Here's how the part is built. I have some questions about the finished solid (model axes, mm). Give positions to 0.01 mm unless a question says otherwise; leave off trailing zeros. Use one line per item in the form item = value.
from build123d import *

# Parameters (mm, degrees)
BOSS_EXTRUDE1_DEPTH  = 3.000000026
SKETCH2_R            = 2.767129072
SKETCH2_R_2          = 3.006829377
BOSS_EXTRUDE2_DEPTH  = 3
M3_CLEARANCE_HOLE1_D = 3.2


with BuildPart() as part:
    # Sketch1 → Boss-Extrude1 (new body)
    with BuildSketch(Plane.XZ):
        Polygon((3.305407241, 0.060769264), (3.999999724, 0), (34.000001848, 0), (34.694589674, 0.060769264), (35.368077457, 0.241229776), (35.99999845, 0.535898609), (36.571152508, 0.935822492), (37.064179778, 1.428849762), (37.464100868, 2.000000095), (37.758767605, 2.631919459), (37.939228117, 3.305407474), (37.999998778, 4.00000019), (37.939228117, 4.694593139), (37.758767605, 5.368080921), (37.464100868, 6.000000052), (37.064179778, 6.571150385), (36.571152508, 7.064177655), (35.99999845, 7.464101538), (35.368077457, 7.758770604), (34.694589674, 7.939230651), (34.000001848, 8.00000038), (3.999999724, 8.00000038), (3.305407241, 7.939230651), (2.631919459, 7.758770604), (1.999998465, 7.464101538), (1.428848132, 7.064177655), (0.935820863, 6.571150385), (0.535897911, 6.000000052), (0.241229311, 5.368080921), (0.060768798, 4.694593139), (0, 4.00000019), (0.060768798, 3.305407474), (0.241229311, 2.631919459), (0.535897911, 2.000000095), (0.935820863, 1.428849762), (1.428848132, 0.935822492), (1.999998465, 0.535898609), (2.631919459, 0.241229776), align=None)
        Polygon((32.391306013, 2.650146373), (32.181344926, 2.950000111), (32.026644796, 3.281757934), (31.931903213, 3.635338973), (31.899999827, 4.00000019), (31.931903213, 4.364661407), (32.026644796, 4.718242679), (32.181344926, 5.050000269), (32.391306013, 5.349854007), (32.650146633, 5.608693697), (32.949998975, 5.818653386), (33.281758428, 5.973354913), (33.635336906, 6.068096496), (34.000001848, 6.099999882), (34.364659339, 6.068096496), (34.718241543, 5.973354913), (35.04999727, 5.818653386), (35.349853337, 5.608693697), (35.608693957, 5.349854007), (35.818651319, 5.050000269), (35.973355174, 4.718242679), (36.068096757, 4.364661407), (36.100000143, 4.00000019), (36.068096757, 3.635338973), (35.973355174, 3.281757934), (35.818651319, 2.950000111), (35.608693957, 2.650146373), (35.349853337, 2.391306916), (35.04999727, 2.181346994), (34.718241543, 2.0266457), (34.364659339, 1.931903884), (34.000001848, 1.900000265), (33.635336906, 1.931903884), (33.281758428, 2.0266457), (32.949998975, 2.181346994), (32.650146633, 2.391306916), align=None, mode=Mode.SUBTRACT)
        Polygon((5.685296841, 2.58586742), (5.414132029, 2.314702375), (5.099999718, 2.094744239), (4.752444103, 1.932676416), (4.38202545, 1.833423041), (3.999999724, 1.800000202), (3.617973067, 1.833423041), (3.247555345, 1.932676416), (2.899998799, 2.094744239), (2.58586742, 2.314702375), (2.314701444, 2.58586742), (2.094743773, 2.900000196), (1.932675019, 3.247555811), (1.833422109, 3.617974231), (1.799998805, 4.00000019), (1.833422109, 4.382026382), (1.932675019, 4.752444569), (2.094743773, 5.100000184), (2.314701444, 5.41413296), (2.58586742, 5.685297772), (2.899998799, 5.905256141), (3.247555345, 6.067323964), (3.617973067, 6.166577339), (3.999999724, 6.200000178), (4.38202545, 6.166577339), (4.752444103, 6.067323964), (5.099999718, 5.905256141), (5.414132029, 5.685297772), (5.685296841, 5.41413296), (5.905255675, 5.100000184), (6.067323498, 4.752444569), (6.166576408, 4.382026382), (6.199999712, 4.00000019), (6.166576408, 3.617974231), (6.067323498, 3.247555811), (5.905255675, 2.900000196), align=None, mode=Mode.SUBTRACT)
    extrude(amount=-BOSS_EXTRUDE1_DEPTH)

    # Sketch2 → Boss-Extrude2 (add)
    with BuildSketch(Plane(origin=(0, 3.000000026, 0), x_dir=(1, 0, 0), z_dir=(0, 1, 0))):
        with Locations((3.930419847, -4.196730993)):
            Circle(SKETCH2_R)
        with Locations((34.148271252, -4.196730993)):
            Circle(SKETCH2_R_2)
    extrude(amount=-BOSS_EXTRUDE2_DEPTH)

    # M3 Clearance Hole1 (through all)
    with Locations(Plane(origin=(0, 3.000000026, 0), x_dir=(1, 0, 0), z_dir=(0, 1, 0))):
        with Locations((3.974411457, -4.108268671), (34.083612048, -4.108268671)):
            Hole(M3_CLEARANCE_HOLE1_D / 2)


solid = part.part
(1) If I drill on probe 1 along X at (y, z) = (0.45, 3); probe 2 along X at (y, z) = (2.55, 4.5); probe 3 along Z at (x, y) = (35, 2.75), over which ranges is the centre line in solid material (lowest first)?
Geometry says:
probe_1 = 0.14 to 2.82, 5.13 to 32.93, 35.24 to 37.86
probe_2 = 0.04 to 2.42, 5.53 to 32.53, 35.63 to 37.96
probe_3 = 0.14 to 2.8, 5.42 to 7.86
(2) Thinking about a two-plate mould opening in Z: for faces 1 (the cylindrical face through (4.18, 1.48, 2.52)), 2 (the flat face through (19, 1, 0)), 3 (the flat face through (19, 3, 4)), which applies, pulls with the +Z half, pulls with the -Z half, needs draft (parallel to the pull), parting line crosses it, or undercut?
Geometry says:
face_1 = undercut
face_2 = pulls with the -Z half
face_3 = needs draft
(3) If we section it at A-A (y = 1.3): Give the number of separate pieces and of enclosed holes in the cut face, plus the area to 3 significant figures.
Geometry says:
separate_pieces = 1
enclosed_holes = 2
area = 274 mm²
